from build123d import *

# Parameters (mm, degrees)
SKETCH_1_W          = 40
SKETCH_1_H          = 5
EXTRUDE_1_DEPTH     = 3
SKETCH_2_W          = 4.5
SKETCH_2_H          = 4
EXTRUDE_2_DEPTH     = 11.5
SKETCH_4_R          = 1
CUT_EXTRUDE_1_DEPTH = 26.024987512
SKETCH_5_W          = 17.1
SKETCH_5_H          = 14.5
SKETCH_5_R          = 1.4
EXTRUDE_3_DEPTH     = 5
EXTRUDE_4_DEPTH     = 3
SKETCH_7_R          = 2.4
SKETCH_7_R_2        = 1.4
EXTRUDE_5_DEPTH     = 0.75
CHAMFER_1_SIZE      = 1
EXTRUDE_11_DEPTH    = 3.99


with BuildPart() as part:
    # Эскиз1 → Бобышка-Вытянуть1 (new body)
    with BuildSketch(Plane.XY):
        Rectangle(SKETCH_1_W, SKETCH_1_H)
    extrude(amount=EXTRUDE_1_DEPTH)

    # Эскиз2 → Бобышка-Вытянуть2 (add)
    with BuildSketch(Plane.XY.offset(3)):
        with Locations((-17.75, -0.5)):
            Rectangle(SKETCH_2_W, SKETCH_2_H)
        with Locations((10.75, -0.5)):
            Rectangle(SKETCH_2_W, SKETCH_2_H)
    extrude(amount=EXTRUDE_2_DEPTH)

    # Эскиз4 → Вырез-Вытянуть1 (cut, through all)
    with BuildSketch(Plane(origin=(0, 1.5, 0), x_dir=(1, 0, 0), z_dir=(0, 1, 0))):
        with Locations(Location((-17.5, -8.75, 0), (0, 0, 270))):
            Circle(SKETCH_4_R)
        with Locations(Location((10.5, -8.75, 0), (0, 0, 90))):
            Circle(SKETCH_4_R)
    extrude(amount=-CUT_EXTRUDE_1_DEPTH, mode=Mode.SUBTRACT)

    # Эскиз5 → Бобышка-Вытянуть3 (add)
    with BuildSketch(Plane.XZ.offset(2.5)):
        with Locations((8.05, 7.25)):
            Rectangle(SKETCH_5_W, SKETCH_5_H)
        with Locations(Location((12.85, 8.75, 0), (0, 0, 83.849360172))):
            Circle(SKETCH_5_R, mode=Mode.SUBTRACT)
    extrude(amount=EXTRUDE_3_DEPTH)

    # Эскиз6 → Бобышка-Вытянуть4 (add)
    with BuildSketch(Plane(origin=(0, 0, 0), x_dir=(-1, 0, 0), z_dir=(0, 0, -1))):
        Polygon((-20, -2.5), (-16.6, -7.5), (-16.6, -2.5), align=None)
        Polygon((20, -2.5), (0.5, -7.5), (0.5, -2.5), align=None)
    extrude(amount=-EXTRUDE_4_DEPTH)

    # Эскиз7 → Бобышка-Вытянуть5 (add)
    with BuildSketch(Plane.XZ.offset(7.5)):
        with Locations(Location((12.85, 8.75, 0), (0, 0, 270))):
            Circle(SKETCH_7_R)
        with Locations(Location((12.85, 8.75, 0), (0, 0, 83.849360172))):
            Circle(SKETCH_7_R_2, mode=Mode.SUBTRACT)
    extrude(amount=EXTRUDE_5_DEPTH)

    # Фаска1
    # the kernel refuses this chamfer: 1 mm, written as the material it adds along each edge
    with BuildSketch(Plane(origin=(12.85, -7.5, 8.75), x_dir=(0, 0, -1), z_dir=(-1, 0, 0))) as chamfer_1_piece_1_section:
        Polygon((2.4 + CHAMFER_1_SIZE, 0), (2.4, CHAMFER_1_SIZE), (2.4, 0), align=None)
    chamfer_1_piece_1 = revolve(axis=Axis((12.85, -7.5, 8.75), (0, -1, 0)), mode=Mode.PRIVATE)
    chamfer_1_piece_1 = split(chamfer_1_piece_1, bisect_by=Plane(origin=(12.85, -8.25, 8.75), z_dir=(0, 1, 0)), keep=Keep.TOP, mode=Mode.PRIVATE)
    add(chamfer_1_piece_1)

    # Эскиз8 → Бобышка-Вытянуть11 (add)
    with BuildSketch(Plane(origin=(0, 1.5, 0), x_dir=(1, 0, 0), z_dir=(0, 1, 0))):
        Polygon((-15.5, -14.5), (-20, -14.5), (-20, -17.5), (13, -17.5), (13, -14.5), align=None)
    extrude(amount=-EXTRUDE_11_DEPTH)


solid = part.part
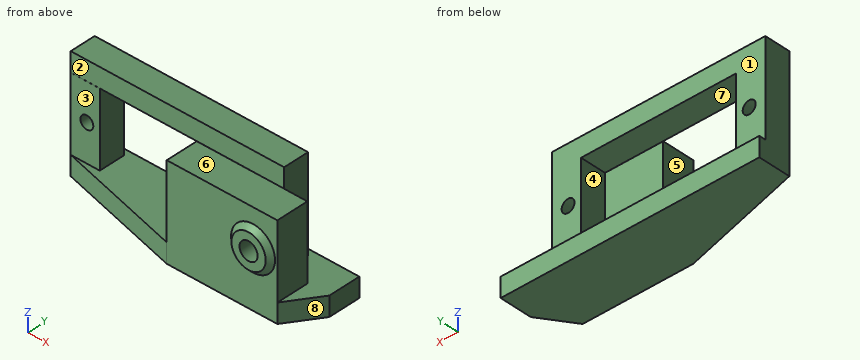
Model file for the job. Use its own axes, mm. Face numbers are marked on the shaded views. A direction names the side the tool comes from. Coordinates: 2 decimals unless noted, no trailing zeros. Order: outer loops, then holes, each group sorted by start corner. A loop starts at its lowest first (then second) coordinate and runs counter-clockwise, first axis right, second up. Notation, with made-up numbers: (33, 51) -> (48, 51) arc R22 cw to (48, 77) -> close; hole circle Ø7 at (28, 64.25). An arc over 180 degrees is marked (long way). Return JSON: item names as keys, results as strings. Group by question number.
Item 1: Tool access for the marked faces 1, 2, 3, 4 and 5: list every direction of +Z, -Z, +X, -X, +Y, -Y with a clear straight run to the whole face (end or side of a thin tool).
Item 2: Saw through at A-A on z = 4.75. Write the cut outline in (x, y), then the cut area to 4 significant figures.
Item 3: Pull direction X, two halves, no side cores. Call the marked faces 6, 7 and 8: pulls with the +X half, pulls with the -X half, needs draft (parallel to the pull), parting line crosses it, or undercut.
Item 4: Saw through at B-B on y = -1.25. Write the cut outline in (x, z).
Item 5: Saw through at D-D on y = -6.75. Write the cut outline in (x, z) (3 decimals).
Item 6: Flat gauge pins, fed straight in: P1, Ø2.5, axis at x = 5.5, y = -6, coming from the +Z side; P2, Ø3.5, axis at x = -10.5, z = 15.5, coming from the -Y side; P3, Ø1.1, axis at x = 15.5, z = 10.5, coming from the +Y side. Where does each tip first touch, or does it go through?
Item 7: Wall check: line 1 along X through (y, z) = (1, 12.75); line 2 along Z through (x, y) = (-7, -2); line 3 along Z through (x, y) = (12.85, -6.65). Give the ranges that are in metal, low to high. Write a range as [from, to].
Values found:
{
 "1": {"face 1": "+Z, +X, -X, +Y", "face 2": "+Z, +X, -X, -Y", "face 3": "+Z, -X, -Y", "face 4": "+Y", "face 5": "+Z, -X, +Y, -Y"},
 "2": {"outline": "(-20, -2.5) -> (-15.5, -2.5) -> (-15.5, 1.5) -> (-20, 1.5) -> close; (-0.5, -7.5) -> (16.6, -7.5) -> (16.6, -2.5) -> (13, -2.5) -> (13, 1.5) -> (8.5, 1.5) -> (8.5, -2.5) -> (-0.5, -2.5) -> close", "area": "121.5 mm2"},
 "3": {"face 6": "needs draft", "face 7": "undercut", "face 8": "pulls with the +X half"},
 "4": {"outline": "(-20, 0) -> (20, 0) -> (20, 3) -> (13, 3) -> (13, 17.5) -> (-20, 17.5) -> close; hole circle Ø2 at (-17.5, 8.75); hole (-15.5, 3) -> (8.5, 3) -> (8.5, 14.5) -> (-15.5, 14.5) -> close; hole circle Ø2 at (10.5, 8.75)"},
 "5": {"outline": "(-3.425, 0) -> (17.11, 0) -> (17.11, 3) -> (16.6, 3) -> (16.6, 14.5) -> (-0.5, 14.5) -> (-0.5, 3) -> (-3.425, 3) -> close; hole circle Ø2.8 at (12.85, 8.75)"},
 "6": {"P1": "stops at z = 14.5", "P2": "stops at y = -2.49", "P3": "stops at y = -2.5"},
 "7": {"line 1": "x = [-20, -15.5], [8.5, 13]", "line 2": "z = [0, 3], [14.5, 17.5]", "line 3": "z = [0, 7.35], [10.15, 14.5]"}
}
